from build123d import *

# Parameters (mm, degrees)
SKETCH1_W           = 203.2
SKETCH1_H           = 101.6
BOSS_EXTRUDE1_DEPTH = 2.54
SKETCH2_W           = 198.12
SKETCH2_H           = 96.52
BOSS_EXTRUDE2_DEPTH = 14.478
SKETCH4_W           = 17.78
SKETCH4_H           = 14.478
SKETCH4_W_2         = 15.24
CUT_EXTRUDE6_DEPTH  = 101.6


with BuildPart() as part:
    # Sketch1 → Boss-Extrude1 (new body)
    with BuildSketch(Plane(origin=(0, 0, 0), x_dir=(1, 0, 0), z_dir=(0, 1, 0))):
        with Locations((-18.181052632, -25.132631579)):
            Rectangle(SKETCH1_W, SKETCH1_H)
    extrude(amount=BOSS_EXTRUDE1_DEPTH)

    # Sketch2 → Boss-Extrude2 (add)
    with BuildSketch(Plane(origin=(0, 2.54, 0), x_dir=(1, 0, 0), z_dir=(0, 1, 0))):
        with Locations((-18.181052632, -25.132631579)):
            Rectangle(SKETCH2_W, SKETCH2_H)
    extrude(amount=BOSS_EXTRUDE2_DEPTH)

    # Sketch4 → Cut-Extrude6 (cut)
    with BuildSketch(Plane(origin=(0, 0, -23.127368421), x_dir=(-1, 0, 0), z_dir=(0, 0, -1))):
        with Locations((-51.160947368, 9.779)):
            Rectangle(SKETCH4_W, SKETCH4_H)
        with Locations((96.159052632, 9.779)):
            Rectangle(SKETCH4_W_2, SKETCH4_H)
    extrude(amount=-CUT_EXTRUDE6_DEPTH, mode=Mode.SUBTRACT)


solid = part.part
The listing builds one solid part. Answer for the finished solid, in the listing's coordinates (mm). A direction names the side the tool comes from. Coordinates: 2 decimals unless noted, no trailing zeros. Write each loop counter-clockwise with the first axis right and the second up, starting at its lowest first coordinate (ties: lowest second). Pieces come first, ordered by that corner, then holes. Notation, with made-up numbers: (82, 88) - (107, 88) arc R26 cw to (107, 125) - close; hole circle Ø7 at (81, -20.5). An arc over 180 degrees is marked (long way). Return JSON: item names as keys, results as strings.
1. Which of the six approach directions +Z, -Z, +X, -X, +Y, -Y give full straight-line access (tool end or side, diameter ignored) to faces 4 (the face through (-117.241, 10, 26)), 5 (the face through (-24, 10, -23.127)), 6 (the face through (60.051, 10, 24)), 7 (the face through (-111, 10, 73.393))?
Final values:
{"face 4": "+Z, -Z, -X, +Y", "face 5": "-Z, +X, -X, +Y", "face 6": "+Z, -Z, +Y", "face 7": "+Z, +X, -X, +Y"}
2. The part is cut by section A-A on y = 8. Determine the outline of the cut face in (x, z), then the cut area to 3 significant figures.
Final values:
{"outline": "(-117.24, -23.13) - (-103.78, -23.13) - (-103.78, 73.39) - (-117.24, 73.39) - close; (-88.54, -23.13) - (42.27, -23.13) - (42.27, 73.39) - (-88.54, 73.39) - close; (60.05, -23.13) - (80.88, -23.13) - (80.88, 73.39) - (60.05, 73.39) - close", "area": "15,900 mm^2"}
3. Consider line 1 along X through (y, z) = (9, 36); line 2 along Z through (x, y) = (16, 13.25); line 3 along Y through (x, z) = (43, -3). Determine where each line is inside the solid, lowest interval first.
Final values:
{"line 1": "-117.24 to -103.78, -88.54 to 42.27, 60.05 to 80.88", "line 2": "-23.13 to 73.39", "line 3": "0 to 2.54"}
4. For a pull along X with two mould halves and no side action, classify faces 1 (the face through (-24, 10, 73.393)), 2 (the face through (80.879, 10, 26)), 3 (the face through (42.271, 10, 24)) as +X half, -X half, draft (parallel to the pull), parting line (faces both ways), or undercut.
Final values:
{"face 1": "draft", "face 2": "+X half", "face 3": "undercut"}
5. Each of these flat-tipped pins is pushed along its axis until it touches: pin 1 Ø3 at (x, y) = (22, 7.5) entering from +Z; pin 2 Ø1 at (y, z) = (8.5, 40) entering from -X; pin 3 Ø2 at (x, z) = (58.5, -9) entering from +Y. Where does it stop, or does it pass through?
Final values:
{"pin 1": "z = 73.39", "pin 2": "x = -117.24", "pin 3": "y = 2.54"}
6. The part is cut by section B-B on z = 43. Determine the outline of the cut face in (x, y), then the cut area to 3 significant figures.
Final values:
{"outline": "(-119.78, 0) - (83.42, 0) - (83.42, 2.54) - (80.88, 2.54) - (80.88, 17.02) - (60.05, 17.02) - (60.05, 2.54) - (42.27, 2.54) - (42.27, 17.02) - (-88.54, 17.02) - (-88.54, 2.54) - (-103.78, 2.54) - (-103.78, 17.02) - (-117.24, 17.02) - (-117.24, 2.54) - (-119.78, 2.54) - close", "area": "2,910 mm^2"}
7. The part is cut by section D-D on x = 51. Determine the outline of the cut face in (y, z).
Final values:
{"outline": "(0, -25.67) - (2.54, -25.67) - (2.54, 75.93) - (0, 75.93) - close"}
8. The part is cut by section C-C on x = 11. Determine the outline of the cut face in (y, z).
Final values:
{"outline": "(0, -25.67) - (2.54, -25.67) - (2.54, -23.13) - (17.02, -23.13) - (17.02, 73.39) - (2.54, 73.39) - (2.54, 75.93) - (0, 75.93) - close"}
